Geometry: final body of the model. Coordinates: model frame, mm. A direction names the side the tool comes from. Give positions to 0.01 mm unless a question says otherwise; leave off trailing zeros. Loops run counter-clockwise (first coordinate to the right, second up) from the corner with the lowest first, then second, coordinate; pieces in that order, holes last. Notation, with made-up numbers: (19, 3) -> (35, 3) arc R10 ccw to (35, 19) -> close; hole circle Ø8 at (82, 37). An arc over 180 degrees is marked (long way). Answer in a Markdown table with one row per item. Add a question column.
1) Section query D-D (x = 8.25). Return the cut outline in (y, z), plus the area to 3 significant figures.
2) Access query for faces 1 (the cylindrical face through (12.1, 1.25, 0.57)), 2 (the cylindrical face through (8.715, 14.539, 2.465)). Directions: +Z, -Z, +X, -X, +Y, -Y. A direction counts if a zero-diameter tool reaches every point of the face in a straight line with its end or side. Return the directions, or none.
3) Section query B-B (y = 16.5). Return the cut outline in (x, z), plus the area to 3 significant figures.
4) Draft query along Y for faces 3 (the cylindrical face through (-8.689, 14.565, 2.465)), 4 (the flat face through (0, 1, 0)), 5 (the flat face through (0, 19.05, 2)). Return one class per face: +Y half, -Y half, draft (parallel to the pull), parting line (faces both ways), or undercut.
5) Section query A-A (z = 2.6). Give the number of separate pieces and of enclosed holes in the cut face, plus the area to 3 significant figures.
6) Section query C-C (y = 6). Return the cut outline in (x, z), plus the area to 3 significant figures.
7) Line query: line 1 (X direction, y = -13.5, z = 2.25); line 2 (X direction, y = -14, z = 1.1); line 3 (Y direction, x = 9.5, z = 1.85). Output: solid intervals per line, ascending. Write a range as from..to.
```python
from build123d import *

# Parameters (mm, degrees)
SKETCH1_W           = 25.4
SKETCH1_H           = 38.1
BOSS_EXTRUDE1_DEPTH = 5
SKETCH2_W           = 3.4
SKETCH2_H           = 30.1
CUT_EXTRUDE1_DEPTH  = 24.434856518
FILLET1_R           = 1.7
FILLET2_R           = 1.7
FILLET3_R           = 1.7
FILLET4_R           = 1.7
FILLET5_R           = 2


with BuildPart() as part:
    # Sketch1 → Boss-Extrude1 (new body)
    with BuildSketch(Plane.XY):
        Rectangle(SKETCH1_W, SKETCH1_H)
    extrude(amount=BOSS_EXTRUDE1_DEPTH)

    # Sketch2 → Cut-Extrude1 (cut, through all)
    with BuildSketch(Plane.XY.offset(5)):
        with Locations((7.5, 0)):
            Rectangle(SKETCH2_W, SKETCH2_H)
        with Locations((-7.5, 0)):
            Rectangle(SKETCH2_W, SKETCH2_H)
    extrude(amount=-CUT_EXTRUDE1_DEPTH, mode=Mode.SUBTRACT)

    # Fillet1
    fillet1_edges = [part.edges().sort_by_distance(p)[0] for p in [
        (-5.8, 15.05, 2.5),
        (-9.2, 15.05, 2.5),
    ]]
    fillet(fillet1_edges, radius=FILLET1_R - 0.0001)  # a hair under: the kernel refuses the full size

    # Fillet2
    fillet2_edges = [part.edges().sort_by_distance(p)[0] for p in [
        (-5.8, -15.05, 2.5),
        (-9.2, -15.05, 2.5),
    ]]
    fillet(fillet2_edges, radius=FILLET2_R - 0.0001)  # a hair under: the kernel refuses the full size

    # Fillet3
    fillet3_edges = [part.edges().sort_by_distance(p)[0] for p in [
        (9.2, 15.05, 2.5),
        (5.8, 15.05, 2.5),
    ]]
    fillet(fillet3_edges, radius=FILLET3_R - 0.0001)  # a hair under: the kernel refuses the full size

    # Fillet4
    fillet4_edges = [part.edges().sort_by_distance(p)[0] for p in [
        (9.2, -15.05, 2.5),
        (5.8, -15.05, 2.5),
    ]]
    fillet(fillet4_edges, radius=FILLET4_R - 0.0001)  # a hair under: the kernel refuses the full size

    # Fillet5
    fillet5_edges = [part.edges().sort_by_distance(p)[0] for p in [
        (-12.7, 0, 5),
        (0, -19.05, 5),
        (12.7, 0, 5),
        (0, -19.05, 0),
        (-12.7, 0, 0),
        (12.7, 0, 0),
        (12.7, -19.05, 2.5),
        (-12.7, -19.05, 2.5),
    ]]
    fillet(fillet5_edges, radius=FILLET5_R)


solid = part.part
```
Evaluation:
| question | item | result |
|---|---|---|
| 1 | outline | (-19.05, 2) arc R2 ccw to (-17.05, 0) -> (-14.88, 0) -> (-14.88, 5) -> (-17.05, 5) arc R2 ccw to (-19.05, 3) -> close; (14.88, 0) -> (19.05, 0) -> (19.05, 5) -> (14.88, 5) -> close |
| 1 | area | 40.0 mm² |
| 2 | face 1 | -Z, +X, +Y, -Y |
| 2 | face 2 | +Z, -Z |
| 3 | outline | (-12.7, 2) arc R2 ccw to (-10.7, 0) -> (10.7, 0) arc R2 ccw to (12.7, 2) -> (12.7, 3) arc R2 ccw to (10.7, 5) -> (-10.7, 5) arc R2 ccw to (-12.7, 3) -> close |
| 3 | area | 124 mm² |
| 4 | face 3 | undercut |
| 4 | face 4 | draft |
| 4 | face 5 | +Y half |
| 5 | separate pieces | 1 |
| 5 | enclosed holes | 2 |
| 5 | area | 766 mm² |
| 6 | outline | (-12.7, 2) arc R2 ccw to (-10.7, 0) -> (-9.2, 0) -> (-9.2, 5) -> (-10.7, 5) arc R2 ccw to (-12.7, 3) -> close; (-5.8, 0) -> (5.8, 0) -> (5.8, 5) -> (-5.8, 5) -> close; (9.2, 0) -> (10.7, 0) arc R2 ccw to (12.7, 2) -> (12.7, 3) arc R2 ccw to (10.7, 5) -> (9.2, 5) -> close |
| 6 | area | 89.6 mm² |
| 7 | line 1 | -12.7..-9.19, -5.81..5.81, 9.19..12.7 |
| 7 | line 2 | -12.49..-9.07, -5.93..5.93, 9.07..12.49 |
| 7 | line 3 | -19.04..19.05 |
